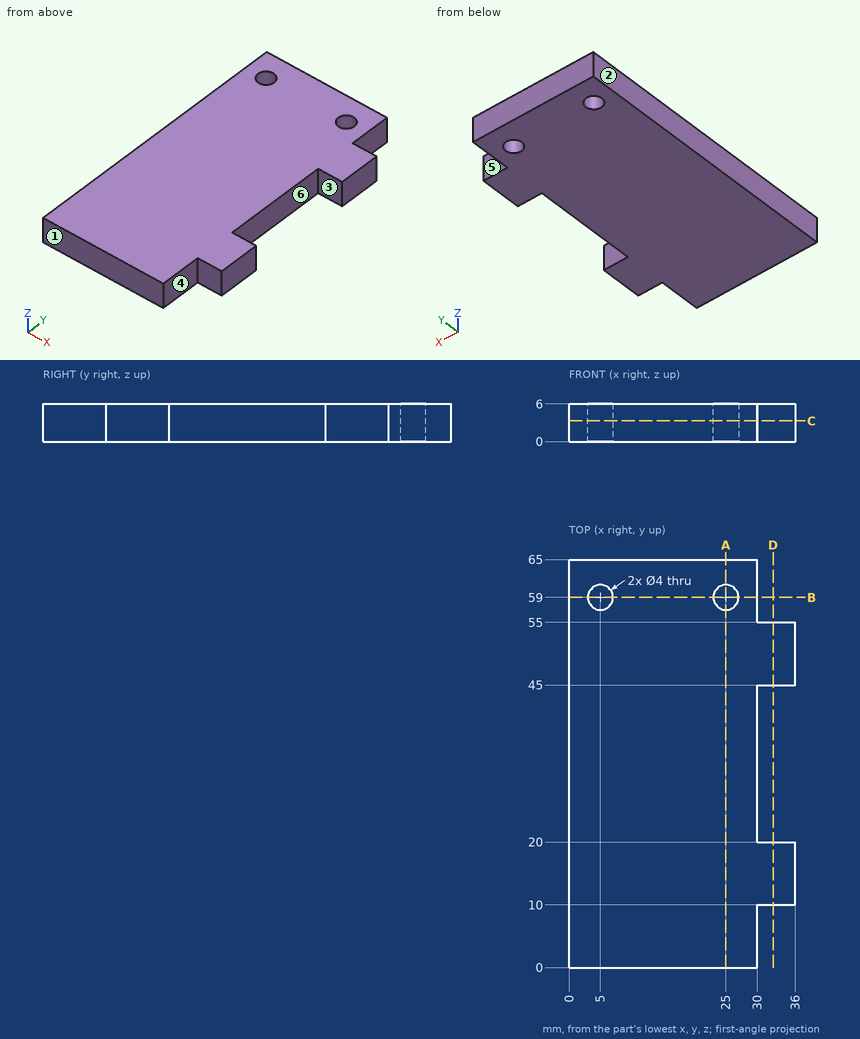
Answer from the drawing. Dimensions are ordinates in mm from the lowest x, y and z of the part. A direction names the side the tool comes from. Round coordinates to 2 decimals unless told otherwise and drop trailing zeros. Order: outer loops, then holes, each group sorted by start corner. A loop starts at its lowest first (then second) coordinate and runs counter-clockwise, first axis right, second up. Notation, with made-up numbers: (-35, 24.5) - (-29, 24.5) arc R29 cw to (-29, 59.5) - close; hole circle Ø8 at (63.5, -8). An arc over 180 degrees is marked (long way). Put each result on its own line as item: value. Start each with the question number.
(1) Given P1, Ø1.8, axis at x = 33, z = 3, coming from the -Y side; P2, Ø3, axis at x = 32.5, z = 2, coming from the +Y side; P3, Ø3, axis at y = 28.5, z = 3, coming from the +X side, each flat-ended and moving along its own axis, determine where each tip first touches the part or whether it passes through.
(2) Find section A-A (x = 25). Give the vertices of the cut face in (y, z).
(3) Find section D-D (x = 32.5). Give the vertices of the cut face in (y, z).
(4) Find section C-C (z = 3.3). Give the vertices of the cut face in (x, y).
(5) Determine the mould class of the marked faces 1, 2 and 3 for opening direction Y: released by +Y, released by -Y, zero draft, split by the parting line, or undercut.
(6) Straight lines are drawn through the part: probe 1 along Y at (x, z) = (5, 2.05); probe 2 along X at (y, z) = (7.5, 3); probe 3 along Y at (x, z) = (3.5, 4.6). For each, find the intervals that lie inside material, in ascending order. Write a range as from..to.
(7) Find section B-B (y = 59). Give the vertices of the cut face in (x, z).
(8) For the marked faces 4, 5 and 6, determine the directions among +Z, -Z, +X, -X, +Y, -Y from which every point of the face is accessible in a straight line to the end or side of a thin tool.
Reply:
1. P1: y = 10
1. P2: y = 55
1. P3: x = 30
2. outline: (0, 0) - (57, 0) - (57, 6) - (0, 6) - close; (61, 0) - (65, 0) - (65, 6) - (61, 6) - close
3. outline: (10, 0) - (20, 0) - (20, 6) - (10, 6) - close; (45, 0) - (55, 0) - (55, 6) - (45, 6) - close
4. outline: (0, 0) - (30, 0) - (30, 10) - (36, 10) - (36, 20) - (30, 20) - (30, 45) - (36, 45) - (36, 55) - (30, 55) - (30, 65) - (0, 65) - close; hole circle Ø4 at (5, 59); hole circle Ø4 at (25, 59)
5. face 1: released by -Y
5. face 2: zero draft
5. face 3: undercut
6. probe 1: 0..57, 61..65
6. probe 2: 0..30
6. probe 3: 0..57.68, 60.32..65
7. outline: (0, 0) - (3, 0) - (3, 6) - (0, 6) - close; (7, 0) - (23, 0) - (23, 6) - (7, 6) - close; (27, 0) - (30, 0) - (30, 6) - (27, 6) - close
8. face 4: +Z, -Z, +X, -Y
8. face 5: +Z, -Z, +X, +Y
8. face 6: +Z, -Z, +X
